Read the model definition and answer for the solid it produces. Units are mm, in the model's axes. A direction names the side the tool comes from. Round coordinates to 2 decimals unless told otherwise and drop trailing zeros. Order: outer loops, then holes, each group sorted by start corner. A loop starts at its lowest first (then second) coordinate and runs counter-clockwise, first axis right, second up. Notation, with made-up numbers: (2, -13.75) - (22, -13.75) arc R8 ccw to (22, -0.75) - close; hole circle Ø9 at (-19, -16). An arc over 180 degrees is marked (long way). One line per question, with ' | ' between items. Start each with the question number.
1) The part is cut by section A-A, the plane x = 0. Give the vertices of the cut face in (y, z), plus the area to 3 significant figures.
2) The part is cut by section D-D, the plane y = 20. Give the vertices of the cut face in (x, z), plus the area to 3 significant figures.
3) The part is cut by section B-B, the plane y = 29.5. Give the vertices of the cut face in (x, z), plus the area to 3 significant figures.
4) Straight lines are drawn through the part: line 1 (Y direction, x = 0, z = 0.5); line 2 (Y direction, x = 7, z = 0.6); line 3 (Y direction, x = 16, z = 1.15). For each, find the intervals that lie inside material, in ascending order. Write a range as from..to.
5) A flat-ended cylindrical pin translates along its axis: pin 1 (1 mm diameter, centred on y = 35, z = 0.5, fed in from -X). Find the tip coordinate at first contact, or state that the pin passes through.
6) For faces 4 (the cylindrical face through (-3.9, 40.86, 1.01)), 5 (the cylindrical face through (3.902, 68.057, 1.014)), 6 (the cylindrical face through (-0.33, 14.42, 1.01)), determine the directions among +Z, -Z, +X, -X, +Y, -Y from which every point of the face is accessible in a straight line to the end or side of a thin tool.
7) The part is cut by section C-C, the plane z = 1.7. Count the separate pieces of the cut face and the enclosed holes in it, plus the area to 3 significant figures.
8) The mould has two halves that part along X. Classify faces 1 (the cylindrical face through (-16.5, 90.82, 0.99)), 2 (the flat face through (7, 68.912, 1)), 3 (the flat face through (10.064, 71.635, 0.986)): pulls with the +X half, pulls with the -X half, needs draft (parallel to the pull), parting line crosses it, or undercut.
Autodesk Inventor part; units mm, degrees
ref_plane "YZ Plane" through (0, 0, 0) normal (1, 0, 0) x (0, 1, 0)
ref_plane "XZ Plane" through (0, 0, 0) normal (0, 1, 0) x (-1, 0, 0)
ref_plane "XY Plane" through (0, 0, 0) normal (0, 0, 1) x (1, 0, 0)
sketch "Sketch1" plane through (0, 0, 0) normal (0, 0, 1) x (1, 0, 0)
  circle A0 centre (-14, 4) radius 1.5
  circle A1 centre (-10, 13) radius 1.5
  circle A2 centre (-7, 4) radius 1.5
  line L0 (-20, 0) -> (-20, 8)
  line L1 (0, 0) -> (-20, 0)
  line L2 (0, 40) -> (0, 0)
  line L3 (-10, 40) -> (0, 40)
  line L4 (-10, 23) -> (-10, 40)
  line L5 (-10, 23) -> (-20, 8)
  circle A3 centre (14, 4) radius 1.5
  circle A4 centre (10, 13) radius 1.5
  circle A5 centre (7, 4) radius 1.5
  line L6 (20, 0) -> (20, 8)
  line L7 (10, 23) -> (20, 8)
  line L8 (10, 23) -> (10, 40)
  line L9 (10, 40) -> (0, 40)
  line L10 (0, 40) -> (0, 0)
  line L11 (0, 0) -> (20, 0)
  line L12 (3, 84.8834) -> (-3, 84.8834)
  line L13 (-3, 84.8834) -> (-3, -165.1166)
  line L14 (3, -165.1166) -> (-3, -165.1166)
  line L15 (3, 84.8834) -> (3, -165.1166)
  circle A6 centre (-9, 80.8834) radius 1.5
  circle A7 centre (-7, 90.8834) radius 1.5
  circle A8 centre (-15, 90.8834) radius 1.5
  line L16 (-12.05, 74.2834) -> (-8.0217, 68.9123)
  line L17 (-8.0217, 68.9123) -> (0, 68.9123)
  line L18 (0, 94.8834) -> (0, 68.9123)
  line L19 (0, 94.8834) -> (-20, 94.8834)
  line L20 (-20, 79.501) -> (-20, 94.8834)
  arc A9 (-12.05, 74.2834) -> (-20, 79.501) centre (-23.25, 65.8834) ccw
  line L21 (3, 94.8834) -> (3, 68.9123)
  circle A10 centre (9, 80.8834) radius 1.5
  circle A11 centre (7, 90.8834) radius 1.5
  circle A12 centre (15, 90.8834) radius 1.5
  line L22 (12.05, 74.2834) -> (8.0217, 68.9123)
  arc A13 (20, 79.501) -> (12.05, 74.2834) centre (23.25, 65.8834) ccw
  line L23 (20, 79.501) -> (20, 94.8834)
  line L24 (0, 94.8834) -> (20, 94.8834)
  line L25 (0, 94.8834) -> (0, 68.9123)
  line L26 (8.0217, 68.9123) -> (0, 68.9123)
  line L27 (-20, 8) -> (20, 8)
  line L28 (-3, 40) -> (3, 40)
  line L29 (3, 40) -> (3, 68.9123)
  line L30 (3, 68.9123) -> (-3, 68.9123)
  line L31 (-3, 68.9123) -> (-3, 40)
  point P0 (3, 40)
  point P1 (-3, 68.9123)
extrude "Extrusion1" add sketch "Sketch1" along normal blind 2 contours L5 L4 L3 L13 L27 | L13 L3 L2 L27 | L13 L17 L26 L15 L9 L3 | L2 L9 L15 L27 | L17 L16 A9 L20 L19 L18 L12 L13 | L13 L12 L18 L17 | L15 L9 L8 L7 L27 | L18 L12 L15 L26 | L15 L21 L24 L23 A13 L22 L26 | L18 L24 L21 L12
chamfer "Chamfer1" distance 5 angle 45 2 edges at (20, 8, 1) (-20, 8, 1)
fillet "Fillet1" radius 3 4 edges at (3, 40, 1) (-3, 40, 1) (-3, 68.9123, 1) (3, 68.9123, 1)
sketch "Sketch2" plane through (0, 0, 2) normal (0, 0, 1) x (1, 0, 0)
  line L0 (-15, 8) -> (-17.2265, 12.1603)
  line L1 (-15, 8) -> (15, 8)
  line L2 (17.2265, 12.1603) -> (15, 8)
  line L3 (17.2265, 12.1603) -> (10, 23)
  line L4 (10, 23) -> (10, 40)
  line L5 (10, 40) -> (6, 40)
  arc A0 (3, 43) -> (6, 40) centre (6, 43) ccw
  line L6 (3, 43) -> (3, 65.9123)
  arc A1 (6, 68.9123) -> (3, 65.9123) centre (6, 65.9123) ccw
  line L7 (6, 68.9123) -> (8.0217, 68.9123)
  line L8 (8.0217, 68.9123) -> (12.05, 74.2834)
  arc A2 (20, 79.501) -> (12.05, 74.2834) centre (23.25, 65.8834) ccw
  line L9 (20, 79.501) -> (20, 94.8834)
  line L10 (20, 94.8834) -> (-20, 94.8834)
  line L11 (-20, 94.8834) -> (-20, 79.501)
  arc A3 (-12.05, 74.2834) -> (-20, 79.501) centre (-23.25, 65.8834) ccw
  line L12 (-12.05, 74.2834) -> (-8.0217, 68.9123)
  line L13 (-8.0217, 68.9123) -> (-6, 68.9123)
  arc A4 (-3, 65.9123) -> (-6, 68.9123) centre (-6, 65.9123) ccw
  line L14 (-3, 65.9123) -> (-3, 43)
  arc A5 (-6, 40) -> (-3, 43) centre (-6, 43) ccw
  line L15 (-6, 40) -> (-10, 40)
  line L16 (-10, 40) -> (-10, 23)
  line L17 (-10, 23) -> (-17.2265, 12.1603)
  circle A6 centre (10, 13) radius 1.5
  circle A7 centre (7, 90.8834) radius 1.5
  circle A8 centre (9, 80.8834) radius 1.5
  circle A9 centre (15, 90.8834) radius 1.5
  circle A10 centre (-9, 80.8834) radius 1.5
  circle A11 centre (-7, 90.8834) radius 1.5
  circle A12 centre (-15, 90.8834) radius 1.5
  circle A13 centre (-10, 13) radius 1.5
  circle A14 centre (7, 90.8834) radius 1.5
  line L18 (7, 90.8834) -> (7, 35.8834)
  line L19 (7, 35.8834) -> (7, 25.8834)
  circle A15 centre (7, 35.8834) radius 1.5
  circle A16 centre (7, 25.8834) radius 1.5
  circle A17 centre (-7, 90.8834) radius 1.5
  line L20 (-7, 90.8834) -> (-7, 35.8834)
  line L21 (-7, 35.8834) -> (-7, 25.8834)
  circle A18 centre (-7, 35.8834) radius 1.5
  circle A19 centre (-7, 25.8834) radius 1.5
  line L22 (-7, 35.8834) -> (7, 35.8834)
  line L23 (-7, 25.8834) -> (7, 25.8834)
  circle A20 centre (0, 35.8834) radius 1.5
  circle A21 centre (0, 25.8834) radius 1.5
  line L24 (0, 25.8834) -> (0, 15.8834)
  circle A22 centre (0, 15.8834) radius 1.5
  line L25 (0, 35.8834) -> (0, 75.8834)
  line L26 (0, 75.8834) -> (0, 85.8834)
  circle A23 centre (0, 85.8834) radius 1.5
  circle A24 centre (0, 75.8834) radius 1.5
  point P0 (0, 0)
  dimension "d6" = 55
  dimension "d7" = 10
  dimension "d8" = 3
  dimension "d9" = 3
  dimension "d10" = 55
  dimension "d11" = 10
  dimension "d12" = 3
  dimension "d13" = 3
  dimension "d14" = 3
  dimension "d15" = 3
  dimension "d16" = 10
  dimension "d17" = 3
  dimension "d18" = 40
  dimension "d19" = 10
  dimension "d20" = 3
  dimension "d21" = 3
extrude "Extrusion2" cut sketch "Sketch2" against normal blind 10 contours A22 | A23 | A24 L26 L25 | L25 L26 A24 | A18 L22 L20 | L20 L21 A18 | L22 A18 L21 | A15 L19 L18 | L18 L22 A15 | A20 L25 L22 | L22 A20 | A19 L23 L21 | L21 L23 A19 | L19 A15 L22 | L25 A20 L22 | A21 L23 | L23 L24 A21 | A16 L23 L19 | L19 L23 A16 | L23 A21 L24
properties part number "body_bone_4"
Values:
1) outline: (8, 0) - (14.38, 0) - (14.38, 2) - (8, 2) - close; (17.38, 0) - (24.38, 0) - (24.38, 2) - (17.38, 2) - close; (27.38, 0) - (34.38, 0) - (34.38, 2) - (27.38, 2) - close; (37.38, 0) - (74.38, 0) - (74.38, 2) - (37.38, 2) - close; (77.38, 0) - (84.38, 0) - (84.38, 2) - (77.38, 2) - close; (87.38, 0) - (94.88, 0) - (94.88, 2) - (87.38, 2) - close | area: 144 mm^2
2) outline: (-12, 0) - (12, 0) - (12, 2) - (-12, 2) - close | area: 48.0 mm^2
3) outline: (-10, 0) - (10, 0) - (10, 2) - (-10, 2) - close | area: 40.0 mm^2
4) line 1: y = 8..14.38, 17.38..24.38, 27.38..34.38, 37.38..74.38, 77.38..84.38, 87.38..94.88 | line 2: y = 8..24.38, 27.38..34.38, 37.38..40, 68.91..89.38, 92.38..94.88 | line 3: y = 9.87..14, 77.86..89.77, 92..94.88
5) pin 1: stops at x = -10
6) face 4: +Z, -Z, -X | face 5: +Z, -Z, +X | face 6: +Z, -Z
7) separate pieces: 1 | enclosed holes: 17 | area: 1,710 mm^2
8) face 1: undercut | face 2: needs draft | face 3: pulls with the +X half
